The listing builds one solid part. Answer for the finished solid, in the listing's coordinates (mm). A direction names the side the tool comes from. Round coordinates to 2 decimals unless told otherwise and drop trailing zeros. Order: outer loops, then holes, each group sorted by start corner. A loop starts at its lowest first (then second) coordinate and runs counter-clockwise, first axis right, second up. Notation, with made-up numbers: M -38,84.5 L 3,84.5 A21 cw 3,122.5 Z; hole C -14.5,-17 d11. An arc over 180 degrees is marked long. Write item = value, one per line. Start each with the question number.
(1) Straight lines are drawn through the part: probe 1 along Z at (x, y) = (-0.1, -2.75); probe 2 along Z at (x, y) = (-2.35, 4.5); probe 3 along X at (y, z) = (-4.5, 1.5). For each, find the intervals that lie inside material, in ascending order. Write a range as from..to.
(2) Which of the six approach directions +Z, -Z, +X, -X, +Y, -Y give full straight-line access (tool end or side, diameter ignored) to faces 1 (the face through (-2.5, -0.1, 0.3)), 2 (the face through (2, 0, 0))?
(3) Each of these flat-tipped pins is pushed along its axis until it touches: pin 1 (1.5 mm diameter, centred on x = -0.5, y = -4, fed in from +Z); pin 2 (3 mm diameter, centred on x = -2, y = 3, fed in from -Z). Where does it stop, or does it pass through?
(4) A cutting plane is placed at A-A, the plane x = 0. Determine the outline of the cut face in (y, z), and give its area (3 significant figures).
(5) For a pull along Z with two mould halves and no side action, classify faces 3 (the face through (-2.5, -0.1, -0.3)), 4 (the face through (2.44, -9.89, 0.1)) as released by +Z, released by -Z, zero draft, split by the parting line, or undercut.
(6) A cutting plane is placed at C-C, the plane z = 0. Determine the outline of the cut face in (x, y).
(7) A cutting plane is placed at B-B, the plane y = 5.5. Determine the outline of the cut face in (x, z), and give its area (3 significant figures).
from build123d import *

# Parameters (mm, degrees)
ESQUISSE1_W                  = 1
ESQUISSE1_H                  = 20
ENL_V_MAT_EXTRU_1_DEPTH      = 11.862780491
ENL_V_MAT_EXTRU_1_DEPTH_BACK = 11.862780491
ESQUISSE2_W                  = 3
ESQUISSE2_H                  = 0.6


with BuildPart() as part:
    # Esquisse1 → Base-Révolution (revolve)
    with BuildSketch(Plane.XY, mode=Mode.PRIVATE) as base_r_volution_sk:
        with Locations((2.5, 0)):
            Rectangle(ESQUISSE1_W, ESQUISSE1_H)
    revolve(base_r_volution_sk.sketch.rotate(Axis((0, 10, 0), (0, -1, 0)), 90), axis=Axis((0, 10, 0), (0, -1, 0)))

    # Chanfrein1: read off the stored shape, not the designer's step
    # Chanfrein1 outline → Chanfrein1 (revolve, cut)
    with BuildSketch(Plane.XY):
        Polygon((3, 10), (2.333333333, 10), (3, 9.333333333), align=None)
        Polygon((3, -10), (3, -9.333333333), (2.333333333, -10), align=None)
    revolve(axis=Axis((0, 0, 0), (0, 1, 0)), mode=Mode.SUBTRACT)

    # Esquisse2 → Enlèv. mat.-Extru.1 (cut, two sides: drawn at the far end of the back side and taken through both)
    with BuildSketch(Plane(origin=(0, 0, 0), x_dir=(-1, 0, 0), z_dir=(0, 1, 0)).offset(-ENL_V_MAT_EXTRU_1_DEPTH_BACK)):
        with Locations((1.5, 0)):
            Rectangle(ESQUISSE2_W, ESQUISSE2_H)
    extrude(amount=ENL_V_MAT_EXTRU_1_DEPTH + ENL_V_MAT_EXTRU_1_DEPTH_BACK, mode=Mode.SUBTRACT)


solid = part.part
Reported:
q1.probe_1 = -3..-2, 2..3
q1.probe_2 = -1.86..-0.3, 0.3..1.86
q1.probe_3 = -2.6..-1.32, 1.32..2.6
q2.face_1 = -X, +Y, -Y
q2.face_2 = +Y, -Y
q3.pin_1 = 3
q3.pin_2 = -2.96
q4.outline = M -10,-2.33 L -9.33,-3 L 9.33,-3 L 10,-2.33 L 10,-2 L -10,-2 Z; M -10,2 L 10,2 L 10,2.33 L 9.33,3 L -9.33,3 L -10,2.33 Z
q4.area = 39.1 mm²
q5.face_3 = undercut
q5.face_4 = split by the parting line
q6.outline = M 2,-10 L 2.33,-10 L 3,-9.33 L 3,9.33 L 2.33,10 L 2,10 Z
q7.outline = M -2.98,-0.3 A3 ccw long -2.98,0.3 L -1.98,0.3 A2 cw long -1.98,-0.3 Z
q7.area = 15.1 mm²
